Print and shaded views of the part. All mm, measured from the part's lowest x, y and z. A direction names the side the tool comes from. Round coordinates to 2 decimals unless told otherwise and drop trailing zeros. Loops run counter-clockwise (first coordinate to the right, second up) from the corner with the lowest first, then second, coordinate; pieces in that order, holes last. Notation, with made-up numbers: (23.25, 50.5) -> (48.25, 50.5) arc R20 ccw to (48.25, 66.5) -> close; hole circle Ø5 at (-1, -3). An arc over 180 degrees is marked (long way). Answer as CSV lines item,"result".
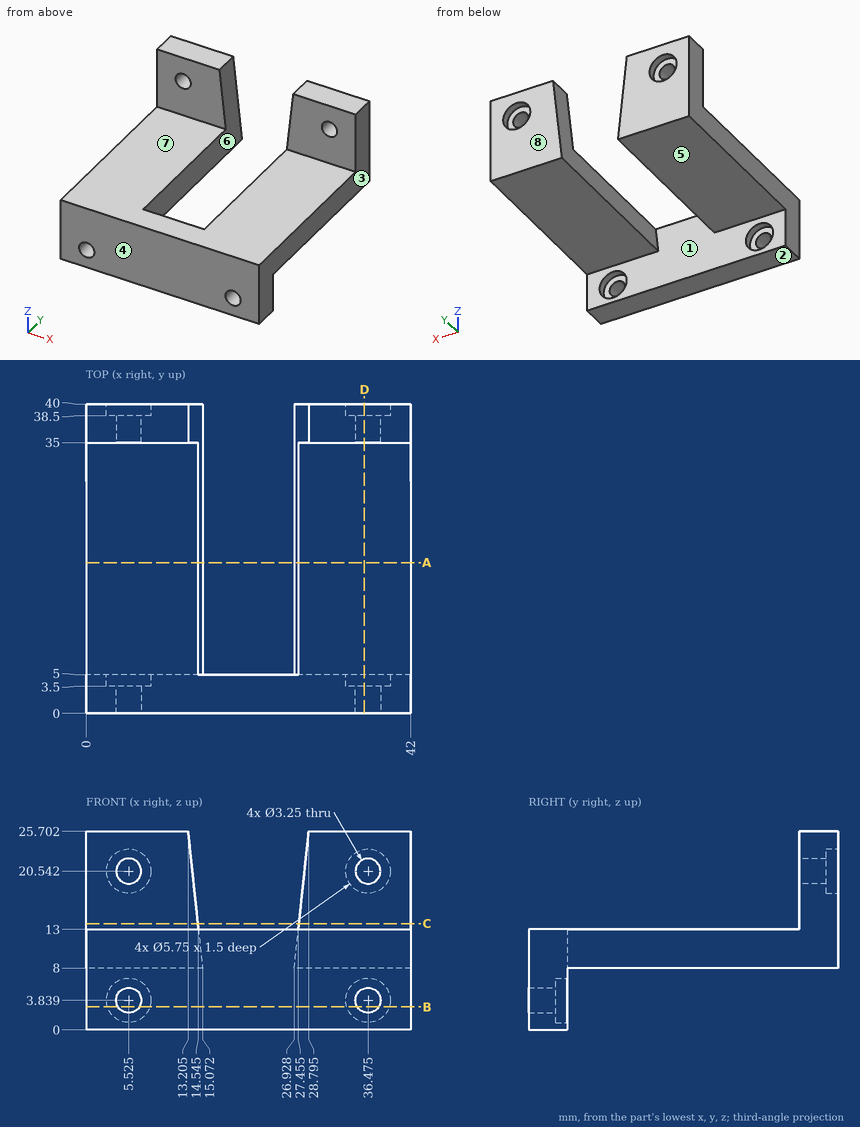
Q1. Two-plate mould, pull along X, no slides. Class the marked faces 1, 2 and 3: pulls with the +X half, pulls with the -X half, needs draft (parallel to the pull), parting line crosses it, or undercut.
Results:
face 1,"undercut"
face 2,"needs draft"
face 3,"pulls with the +X half"
Q2. Tool access for the marked faces 4, 5, 6, 7 and 8: list every direction of +Z, -Z, +X, -X, +Y, -Y with a clear straight run to the whole face (end or side of a thin tool).
Results:
face 4,"+Z, -Z, +X, -X, -Y"
face 5,"-Z, +X, -X, +Y"
face 6,"+Z, +Y"
face 7,"+Z, +X, -X, -Y"
face 8,"+Z, -Z, +X, -X, +Y"
Q3. Drop flat-ended pins along their axis: pin 1 Ø5 at (x, z) = (5.52, 3.84) entering from -Y; pin 2 Ø4.5 at (x, z) = (36.5, 21) entering from +Y; pin 3 Ø7.5 at (x, y) = (5.5, 17) entering from -Z; pin 4 Ø1.7 at (x, z) = (37, 2.5) entering from +Y. Give the stop position or say it passes through.
Results:
pin 1,"y = 0"
pin 2,"y = 38.5"
pin 3,"z = 8"
pin 4,"y = 3.5"
Q4. Slice it at D-D, the plane x = 36. Give the cut face in (y, z) (1 decimal), and give its area (3 significant figures).
Results:
outline,"(0, 0) -> (5, 0) -> (5, 1) -> (3.5, 1) -> (3.5, 2.3) -> (0, 2.3) -> close; (0, 5.4) -> (3.5, 5.4) -> (3.5, 6.7) -> (5, 6.7) -> (5, 8) -> (40, 8) -> (40, 17.7) -> (38.5, 17.7) -> (38.5, 19) -> (35, 19) -> (35, 13) -> (0, 13) -> close; (35, 22.1) -> (38.5, 22.1) -> (38.5, 23.4) -> (40, 23.4) -> (40, 25.7) -> (35, 25.7) -> close"
area,"265 mm2"
Q5. Slice it at B-B, the plane z = 3. Give the cut face in (x, y) (1 decimal), and give its area (3 significant figures).
Results:
outline,"(0, 0) -> (4.1, 0) -> (4.1, 3.5) -> (2.8, 3.5) -> (2.8, 5) -> (0, 5) -> close; (6.9, 0) -> (35.1, 0) -> (35.1, 3.5) -> (33.7, 3.5) -> (33.7, 5) -> (8.3, 5) -> (8.3, 3.5) -> (6.9, 3.5) -> close; (37.9, 0) -> (42, 0) -> (42, 5) -> (39.2, 5) -> (39.2, 3.5) -> (37.9, 3.5) -> close"
area,"174 mm2"
Q6. Slice it at A-A, the plane y = 19.5. Give the cut face in (x, z) (1 decimal).
Results:
outline,"(0, 8) -> (15.1, 8) -> (14.5, 13) -> (0, 13) -> close; (26.9, 8) -> (42, 8) -> (42, 13) -> (27.5, 13) -> close"
Q7. Slice it at C-C, the plane z = 13.75. Give the cut face in (x, y) (1 decimal), and give its area (3 significant figures).
Results:
outline,"(0, 35) -> (14.5, 35) -> (14.5, 40) -> (0, 40) -> close; (27.5, 35) -> (42, 35) -> (42, 40) -> (27.5, 40) -> close"
area,"145 mm2"
Q8. Probe L1, parallel to Y at x = 34, z = 20; L2, parallel to Z at x = 32.5, y = 37.5; L3, parallel to Y at x = 13.5, z = 19. List the from-to ranges inside material, lowest first. Write a range as [from, to].
Results:
L1,"[35, 38.5]"
L2,"[8, 25.7]"
L3,"[35, 40]"
